from build123d import *

# Parameters (mm, degrees)
PAD001_DEPTH = 10
SKETCH_W     = 59
SKETCH_H     = 10
PAD_DEPTH    = 2


with BuildPart() as pad001:
    # Sketch001 → Pad001 (new body)
    with BuildSketch(Plane.XY):
        Polygon((0, 0), (0, -8.4), (2.6, -8.4), (2.6, -7.5), (1.1, -7.5), (1.1, -5.5), (2.6, -5.5), (2.6, -1.5), (56.4, -1.5), (56.4, -5.5), (57.9, -5.5), (57.9, -7.5), (56.4, -7.5), (56.4, -8.4), (59, -8.4), (59, 0), align=None)
    extrude(amount=PAD001_DEPTH)


with BuildPart() as fusion:
    # Sketch → Pad (new body)
    with BuildSketch(Plane.XY):
        with Locations((29.5, -5)):
            Rectangle(SKETCH_W, SKETCH_H)
    extrude(amount=PAD_DEPTH)

    # Fusion: union Pad001
    add(pad001.part)


solid = fusion.part
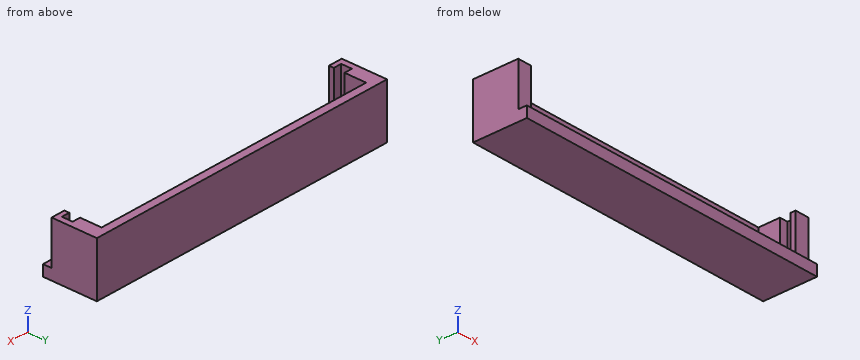
CAD build for the part. Positions are in the model's coordinates, mm. Give positions to 0.01 mm unless a question says otherwise; leave off trailing zeros. Write each loop counter-clockwise with the first axis right and the second up, starting at its lowest first coordinate (ties: lowest second). Pieces come first, ordered by that corner, then holes. Notation, with made-up numbers: M 11.5,-29 L 70.5,-29 A33 ccw 70.5,8 Z; hole C 13.5,29.5 d1. An arc over 180 degrees is marked long. Put each result on its own line as item: value. Start each with the question number.
(1) Band-saw the part on A-A, the plane y = -6. Write the cut outline in (x, z), and give its area (3 significant figures).
(2) Band-saw the part on D-D, the plane y = -2.5. Write the cut outline in (x, z).
(3) Band-saw the part on C-C, the plane z = 4. Write the cut outline in (x, y), and give its area (3 significant figures).
(4) Probe L1, parallel to X at y = -4.5, z = 7.5; L2, parallel to X at y = -7, z = 7.5; L3, parallel to Z at x = 5.5, y = -4. List the from-to ranges inside material, lowest first.
(5) Band-saw the part on B-B, the plane x = 12.5. Write the cut outline in (y, z).
(6) Flat gauge pins, fed straight in: pin 1 Ø3 at (y, z) = (-9, 6) entering from -X; pin 2 Ø2 at (x, z) = (57.5, 7) entering from -Y; pin 3 Ø5 at (x, z) = (47.5, 8) entering from -Y; pin 4 Ø4 at (x, y) = (32, -7.5) entering from +Z. Where does each tip first touch, or does it go through?
Response values:
1. outline: M 0,0 L 59,0 L 59,10 L 57.9,10 L 57.9,2 L 1.1,2 L 1.1,10 L 0,10 Z
1. area: 136 mm2
2. outline: M 0,0 L 59,0 L 59,10 L 56.4,10 L 56.4,2 L 2.6,2 L 2.6,10 L 0,10 Z
3. outline: M 0,-8.4 L 2.6,-8.4 L 2.6,-7.5 L 1.1,-7.5 L 1.1,-5.5 L 2.6,-5.5 L 2.6,-1.5 L 56.4,-1.5 L 56.4,-5.5 L 57.9,-5.5 L 57.9,-7.5 L 56.4,-7.5 L 56.4,-8.4 L 59,-8.4 L 59,0 L 0,0 Z
3. area: 118 mm2
4. L1: x = 0 to 2.6, 56.4 to 59
4. L2: x = 0 to 1.1, 57.9 to 59
4. L3: z = 0 to 2
5. outline: M -10,0 L 0,0 L 0,10 L -1.5,10 L -1.5,2 L -10,2 Z
6. pin 1: stops at x = 0
6. pin 2: stops at y = -8.4
6. pin 3: stops at y = -1.5
6. pin 4: stops at z = 2
